from build123d import *

# Parameters (mm, degrees)
SKETCH1_R           = 4.7625
BOSS_EXTRUDE1_DEPTH = 3.175


with BuildPart() as part:
    # Sketch1 → Boss-Extrude1 (new, symmetric)
    with BuildSketch(Plane(origin=(0, 0, 0), x_dir=(0, 0, -1), z_dir=(1, 0, 0))):
        with BuildLine():
            Line((30, 15), (-1.760727799, 8.072716015))
            ThreePointArc((-1.760727799, 8.072716015), (-8.2625, 0), (-1.760727799, -8.072716015))
            Line((-1.760727799, -8.072716015), (30, -15))
            Line((30, -15), (470, -15))
            Line((470, -15), (501.760727799, -8.072716015))
            ThreePointArc((501.760727799, -8.072716015), (508.2625, 0), (501.760727799, 8.072716015))
            Line((501.760727799, 8.072716015), (470, 15))
            Line((470, 15), (30, 15))
        make_face()
        Circle(SKETCH1_R, mode=Mode.SUBTRACT)
        with Locations(Location((500, 0, 0), (0, 0, 180))):
            Circle(SKETCH1_R, mode=Mode.SUBTRACT)
    extrude(amount=BOSS_EXTRUDE1_DEPTH, both=True)


solid = part.part
Work out the finished part from the listing and answer in its coordinate system (mm). Coordinates: 2 decimals unless noted, no trailing zeros. Order: outer loops, then holes, each group sorted by start corner. A loop starts at its lowest first (then second) coordinate and runs counter-clockwise, first axis right, second up. Notation, with made-up numbers: (19.5, -36.75) - (48.5, -36.75) arc R22 cw to (48.5, 2.25) - close; hole circle Ø11 at (-9, 67.25). An arc over 180 degrees is marked (long way). Put each result on its own line as item: value. Start each with the question number.
1) Flat-ended cylindrical pins translate along their axes: pin 1 (5.5 mm diameter, centred on y = 0, z = -500, fed in from +X); pin 2 (12.5 mm diameter, centred on y = 0, z = 0, fed in from -X) (3 decimals). Find the tip coordinate at first contact, or state that the pin passes through.
2) Find section A-A (y = 0). Give the vertices of the cut face in (x, z) (1 decimal).
3) For a pull along Y with two mould halves and no side action, classify faces 1 (the cylindrical face through (-0.044, -1.431, -495.457)), 2 (the flat face through (-3.175, 0, -246)) as released by +Y, released by -Y, zero draft, split by the parting line, or undercut.
4) Find section B-B (x = 0.75). Give the vertices of the cut face in (y, z) (1 decimal), plus the area to 3 significant figures.
5) Find the intervals of material crossed by line 1 (Z direction, x = -2, y = 3.75); line 2 (Z direction, x = -2.5, y = 3.5); line 3 (Y direction, x = -1.25, z = 0), in increasing order. Write a range as from..to.
Results list:
1. pin 1: passes through
1. pin 2: stops at x = -3.175
2. outline: (-3.2, -508.3) - (3.2, -508.3) - (3.2, -504.8) - (-3.2, -504.8) - close; (-3.2, -495.2) - (3.2, -495.2) - (3.2, -4.8) - (-3.2, -4.8) - close; (-3.2, 4.8) - (3.2, 4.8) - (3.2, 8.3) - (-3.2, 8.3) - close
3. face 1: undercut
3. face 2: zero draft
4. outline: (-15, -470) - (-8.1, -501.8) arc R8.3 ccw to (8.1, -501.8) - (15, -470) - (15, -30) - (8.1, 1.8) arc R8.3 ccw to (-8.1, 1.8) - (-15, -30) - close; hole circle Ø9.5 at (0, -500); hole circle Ø9.5 at (0, 0)
4. area: 14,700 mm^2
5. line 1: z = -507.36..-502.94, -497.06..-2.94, 2.94..7.36
5. line 2: z = -507.48..-503.23, -496.77..-3.23, 3.23..7.48
5. line 3: y = -8.46..-4.76, 4.76..8.46
